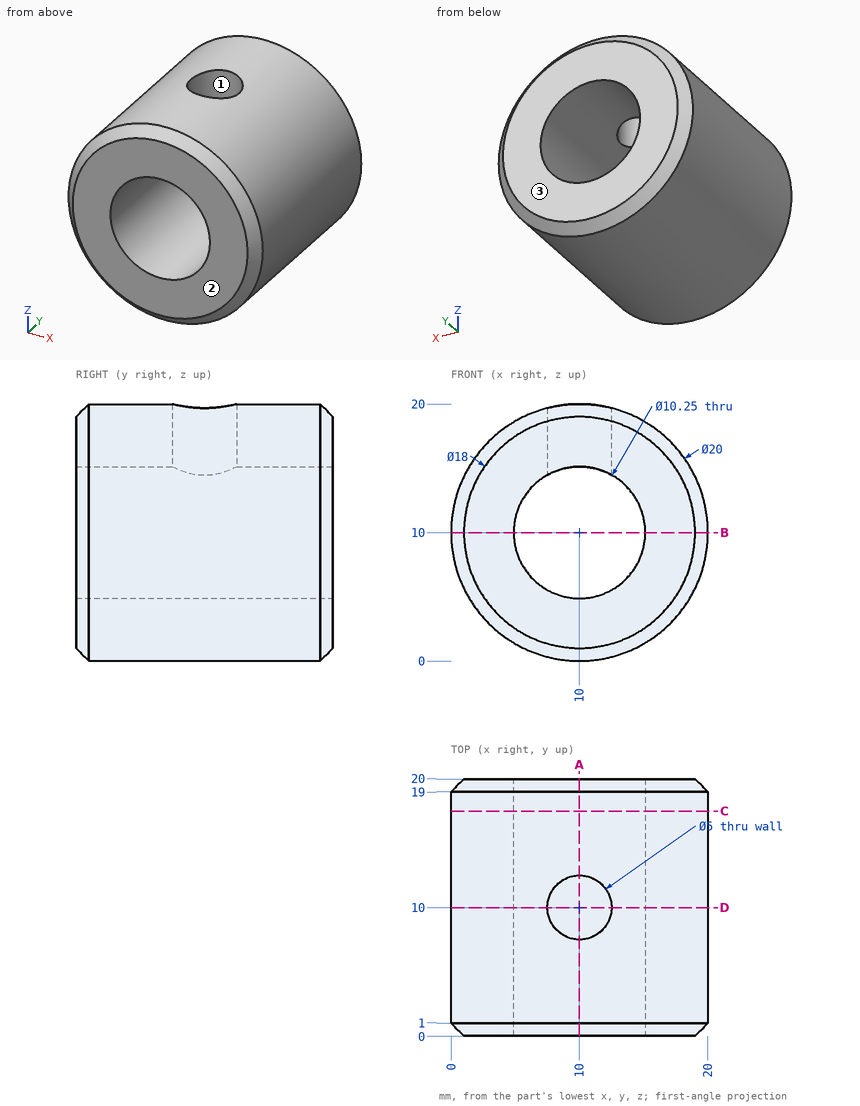
For this review, use the dimensioned drawing (mm, ordinates from the lowest corner) and the shaded views. Round coordinates to 2 decimals unless told otherwise and drop trailing zeros. Order: outer loops, then holes, each group sorted by start corner. A loop starts at its lowest first (then second) coordinate and runs counter-clockwise, first axis right, second up. Notation, with made-up numbers: M 17,8 L 56,8 A28 ccw 56,46 Z; hole C 60,57.25 d1. An arc over 180 degrees is marked long. Use a Markdown table: item, result. Add a question column.
Item 1: Add section B-B, the plane z = 10. Give the boundary of the cut face in (x, y) (3 decimals).
Item 2: Add section A-A, the plane x = 10. Give the boundary of the cut face in (y, z) (3 decimals).
Item 3: Insertion check: pin 1 (12 mm diameter, centred on y = 6, z = 11.5, fed in from -X); pin 2 (1.5 mm diameter, centred on x = 15, y = 8, fed in from -Z); pin 3 (3 mm diameter, centred on x = 15.5, y = 8.5, fed in from -Z); pin 4 (3 mm diameter, centred on y = 10.5, z = 16, fed in from -X). Each pin has a flat end and moves straight along its axis. Give the tip position at first contact, or say it passes through.
Item 4: Add section C-C, the plane y = 17.5. Give the boundary of the cut face in (x, z) (3 decimals).
Item 5: Mouldability with a two-part tool opening along Y and no side actions: class the marked faces 1, 2 and 3 as released by +Y, released by -Y, zero draft, split by the parting line, or undercut.
Item 6: To check wall thickness, follow line 1 along Z through (x, y) = (10, 13) (3 decimals); line 2 along Y through (x, z) = (10, 16.55); line 3 along Z through (x, y) = (5.5, 7.25). State the ranges of each line that lie inside material, in increasing order.
Item 7: Add section D-D, the plane y = 10. Give the boundary of the cut face in (x, z) (3 decimals).
Geometry results:
| question | item | result |
|---|---|---|
| 1 | outline | M 0,1 L 1,0 L 4.875,0 L 4.875,20 L 1,20 L 0,19 Z; M 15.125,0 L 19,0 L 20,1 L 20,19 L 19,20 L 15.125,20 Z |
| 2 | outline | M 0,1 L 1,0 L 19,0 L 20,1 L 20,4.875 L 0,4.875 Z; M 0,15.125 L 7.5,15.125 L 7.5,20 L 1,20 L 0,19 Z; M 12.5,15.125 L 20,15.125 L 20,19 L 19,20 L 12.5,20 Z |
| 3 | pin 1 | stops at x = 0 |
| 3 | pin 2 | stops at z = 0.95 |
| 3 | pin 3 | stops at z = 0.83 |
| 3 | pin 4 | stops at x = 1.07 |
| 4 | outline | C 10,10 d20; hole C 10,10 d10.25 |
| 5 | face 1 | undercut |
| 5 | face 2 | released by -Y |
| 5 | face 3 | released by +Y |
| 6 | line 1 | z = 0 to 4.875, 15.125 to 20 |
| 6 | line 2 | y = 0 to 7.5, 12.5 to 20 |
| 6 | line 3 | z = 1.07 to 7.55, 12.45 to 18.93 |
| 7 | outline | M 7.5,14.474 L 7.5,19.682 A10 ccw long 12.5,19.682 L 12.5,14.474 A5.125 cw long Z |
